Geometry check sheet. Reference: the model listing, model coordinates, mm. Face numbers are marked on the shaded views. A direction names the side the tool comes from. Round coordinates to 2 decimals unless told otherwise and drop trailing zeros. Order: outer loops, then holes, each group sorted by start corner. A loop starts at its lowest first (then second) coordinate and runs counter-clockwise, first axis right, second up.
(1) Go/stop test with flat-tipped pins: pin 1 (6 mm diameter, centred on y = 7.5, z = 4, fed in from -X); pin 2 (4 mm diameter, centred on y = 16.5, z = -11, fed in from -X); pin 3 (2 mm diameter, centred on y = 21, z = 9.5, fed in from +X). Record where each tip stops, or that it passes through.
(2) Material ranges on line 1 along Z through (x, y) = (-11, 26); line 2 along X through (y, z) = (26, 5.75); line 3 along X through (y, z) = (3, -8.75), recorded low to high.
(3) Sectioned sample at D-D (z = -9.5). Record the boundary of the cut face in (x, y), plus the area to 3 significant figures.
(4) Sectioned sample at C-C (x = -6). Record the boundary of the cut face in (y, z).
(5) Release check for a two-part mould opening along Z. For the marked faces 1, 2 and 3 record: +Z half, -Z half, draft (parallel to the pull), parting line (faces both ways), or undercut.
(6) Sectioned sample at B-B (y = 13). Record the boundary of the cut face in (x, z), plus the area to 3 significant figures.
(7) Set-up check for the marked faces 4, 5 and 6: record each of +Z, -Z, +X, -X, +Y, -Y from which the full face is reachable in a straight line by a thin tool's end or side.
(8) Sectioned sample at A-A (x = 13). Record the boundary of the cut face in (y, z), plus the area to 3 significant figures.
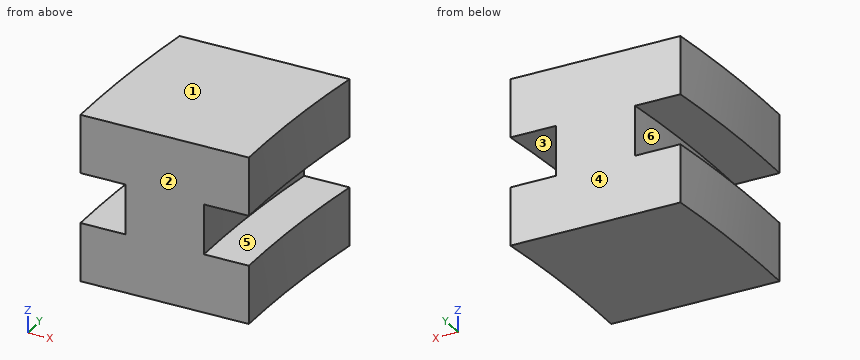
Autodesk Inventor part; units mm, degrees
ref_plane "YZ Plane" through (0, 0, 0) normal (1, 0, 0) x (0, 1, 0)
ref_plane "XY Plane" through (0, 0, 0) normal (0, 0, 1) x (1, 0, 0)
sketch "Sketch1" plane through (0, 0, 0) normal (0, 0, 1) x (1, 0, 0)
  arc A0 (440, 0) -> (0, 0) centre (220, 0) ccw
  dimension "d1" = 440
  dimension "d17" = 220
sketch "Sketch2" plane through (0, 0, 0) normal (0, 1, 0) x (-1, 0, 0)
  line L0 (15, 15) -> (-15, 15)
  line L1 (-15, -15) -> (15, -15)
  line L2 (15, 4.5) -> (7, 4.5)
  line L3 (7, 4.5) -> (7, -4.5)
  line L4 (7, -4.5) -> (15, -4.5)
  line L5 (-15, 4.5) -> (-7, 4.5)
  line L6 (-7, 4.5) -> (-7, -4.5)
  line L7 (-7, -4.5) -> (-15, -4.5)
  line L8 (15, -15) -> (15, -4.5)
  line L9 (15, 4.5) -> (15, 15)
  line L10 (-15, 15) -> (-15, 4.5)
  line L11 (-15, -4.5) -> (-15, -15)
  point P0 (0, 0)
  dimension "d18" = 9
  dimension "d19" = 8
  dimension "d21" = 14
  dimension "d22" = 30
  dimension "d23" = 15
  dimension "d24" = 4.5
  dimension "d25" = 7
sweep "Sweep1" add profiles "Sketch2" path "Sketch1"
sketch "Sketch4" plane through (-15, 0, 15) normal (0, 0, 1) x (1, 0, 0)
  line L0 (470, 0) -> (440, 0)
  line L1 (470, 0) -> (51.3779, 0)
  line L2 (51.3779, 0) -> (51.3779, 30)
  line L3 (51.3779, 30) -> (0.5743, 30)
  line L4 (0.5743, 30) -> (0.5743, 269.0711)
  line L5 (0.5743, 269.0711) -> (470, 269.0711)
  line L6 (470, 269.0711) -> (470, 0)
  point P0 (15, 0)
  dimension "d34" = 469.4257
  dimension "d35" = 30
  dimension "d36" = 50.8036
  dimension "d37" = 269.0711
extrude "Extrusion2" cut sketch "Sketch4" against normal through all
properties part number "LightRail01"
Answer below:
1. pin 1: stops at x = -14.96
1. pin 2: stops at x = -14.55
1. pin 3: stops at x = 16.18
2. line 1: z = -15 to -4.5, 4.5 to 15
2. line 2: x = -13.56 to 16.66
2. line 3: x = -14.98 to 15.02
3. outline: (-15, 0) - (15, 0) arc R205 cw to (17.21, 30) - (-13.08, 30) arc R235 ccw to start
3. area: 903 mm2
4. outline: (0, -15) - (30, -15) - (30, -4.5) - (21.28, -4.5) - (21.28, 4.5) - (30, 4.5) - (30, 15) - (0, 15) - close
5. face 1: +Z half
5. face 2: draft
5. face 3: undercut
6. outline: (-14.64, -15) - (15.41, -15) - (15.41, -4.5) - (7.4, -4.5) - (7.4, 4.5) - (15.41, 4.5) - (15.41, 15) - (-14.64, 15) - (-14.64, 4.5) - (-6.63, 4.5) - (-6.63, -4.5) - (-14.64, -4.5) - close
6. area: 757 mm2
7. face 4: +Z, -Z, +X, -X, +Y
7. face 5: +X, -Y
7. face 6: -X, +Y
8. outline: (0, -15) - (30, -15) - (30, -4.5) - (0, -4.5) - close; (0, 4.5) - (30, 4.5) - (30, 15) - (0, 15) - close
8. area: 630 mm2
